```python
from build123d import *

# Parameters (mm, degrees)
F0_W     = 16
F0_H     = 10
F1_DEPTH = 30
F2_W     = 16
F2_H     = 7
F3_DEPTH = 8
F4_W     = 3.9
F4_H     = 5.5
F5_DEPTH = 8.4
F6_R     = 1.75
F7_DEPTH = 5
F8_F1_R  = 1
F8_F2_R  = 1
F8_F3_R  = 0.9999


# Not quite as in the source:
# - a fillet or chamfer is up to 0.001 mm smaller than in the source, because OpenCascade refuses the exact size
# - a feature names something its author has since deleted; it is built from what else it names


with BuildPart() as f1:
    # F0 (on Top) → F1 (new body)
    with BuildSketch(Plane.XY):
        Rectangle(F0_W, F0_H)
    extrude(amount=F1_DEPTH)

    # F2 (on face) → F3 (cut)
    with BuildSketch(Plane.XY.offset(30)):
        with Locations((0, -1.5)):
            Rectangle(F2_W, F2_H)
    extrude(amount=-F3_DEPTH, mode=Mode.SUBTRACT)

    # F4 (on face) → F5 (cut)
    with BuildSketch(Plane.XY.offset(22)):
        with Locations((-6.05, -0.75)):
            Rectangle(F4_W, F4_H)
        with Locations((6.05, -0.75)):
            Rectangle(F4_W, F4_H)
    extrude(amount=-F5_DEPTH, mode=Mode.SUBTRACT)

    # F6 (on face) → F7 (cut)
    with BuildSketch(Plane.XY.offset(22)):
        with Locations((0, -0.75)):
            Circle(F6_R)
    extrude(amount=-F7_DEPTH, mode=Mode.SUBTRACT)

    # F8: fillet of radius 1 on 13 edges, made by hand

    # F8_f1
    f8_f1_edges = [f1.edges().sort_by_distance(p)[0] for p in [
        (-4.1, -3.5, 17.8),
    ]]
    fillet(f8_f1_edges, radius=F8_F1_R)

    # F8_f2
    f8_f2_edges = [f1.edges().sort_by_distance(p)[0] for p in [
        (4.1, -0.75, 22),
        (-4.1, -0.25, 22),
        (6.05, -3.5, 22),
        (8, 3.5, 30),
        (-8, 3.5, 30),
        (0, 2, 30),
        (0, 5, 30),
        (-8, 2, 21.8),
        (8, 2, 21.8),
        (-4.3928932188, -3.2071067812, 22),
    ]]
    fillet(f8_f2_edges, radius=F8_F2_R)

    # F8_f3 (radius 1 in the source; OpenCascade refuses exactly that, so slightly less here)
    f8_f3_edges = [f1.edges().sort_by_distance(p)[0] for p in [
        (4.1, 2, 17.3),
        (-4.1, 2, 17.3),
        (0, 2, 22),
        (3.8071067812, 2, 21.7071067812),
        (-3.8071067812, 2, 21.7071067812),
    ]]
    fillet(f8_f3_edges, radius=F8_F3_R)


solid = f1.part
```
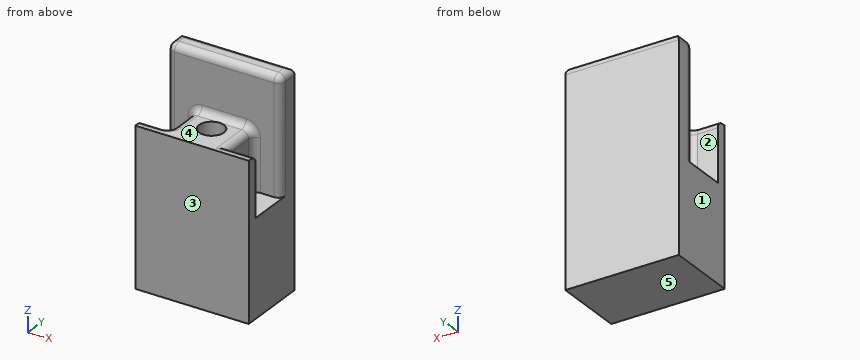
Source: CAD feature listing. Evaluate the final solid. Frame: model axes, mm. Face numbers are marked on the shaded views. A direction names the side the tool comes from. Round coordinates to 2 decimals unless told otherwise and drop trailing zeros. Loops run counter-clockwise (first coordinate to the right, second up) from the corner with the lowest first, then second, coordinate; pieces in that order, holes last. Notation, with made-up numbers: M -38.5,-24 L -0.5,-24 A12 ccw -0.5,-9 Z; hole C -12.75,-6 d9. An arc over 180 degrees is marked long. Use a Markdown table: item, result. Add a question column.
1. Section query A-A on y = -0.75. Return the cut outline in (x, z).
2. Reachability of the marked faces 4 and 5 from +Z, -Z, +X, -X, +Y, -Y: full face, straight path, thin tool, end or side. Return the list, or none.
3. Mould query, pull axis Y, two halves, no side actions, for the marked faces 1, 2 and 3. Classes: pulls with the +Y half, pulls with the -Y half, needs draft (parallel to the pull), parting line crosses it, or undercut.
4. Section query C-C on z = 24.25. Return the cut outline in (x, y), then the cut area to 3 significant figures.
5. Section query D-D on y = 1.5. Return the cut outline in (x, z), then the cut area to 3 significant figures.
6. Contact query for flat-ended pins moving along their axis: P1, Ø5, axis at x = 1, y = -2, coming from the +Z side; P2, Ø3, axis at x = 5, y = -1, coming from the +Z side; P3, Ø1.1, axis at y = 0, z = 16.5, coming from the -X side. Output: stop coordinate, or through.
7. Line query: line 1 (Y direction, x = -7, z = 20.75); line 2 (Y direction, x = 0, z = 18.95); line 3 (Z direction, x = 3, y = -0.25). Output: solid intervals per line, ascending.
Reported:
| question | item | result |
|---|---|---|
| 1 | outline | M -8,0 L 8,0 L 8,13.6 L 4.1,13.6 L 4.1,21 A1 ccw 3.1,22 L 1.75,22 L 1.75,17 L -1.75,17 L -1.75,22 L -3.1,22 A1 ccw -4.1,21 L -4.1,13.6 L -8,13.6 Z |
| 2 | face 4 | +Z, +X, -X, -Y |
| 2 | face 5 | -Z, +X, -X, +Y, -Y |
| 3 | face 1 | needs draft |
| 3 | face 2 | undercut |
| 3 | face 3 | pulls with the -Y half |
| 4 | outline | M -8,3 A1 ccw -7,2 L 7,2 A1 ccw 8,3 L 8,5 L -8,5 Z |
| 4 | area | 47.6 mm² |
| 5 | outline | M -8,0 L 8,0 L 8,13.6 L 4.23,13.6 L 4.23,21 A1.13 ccw 3.1,22.13 L -3.1,22.13 A1.13 ccw -4.23,21 L -4.23,13.6 L -8,13.6 Z |
| 5 | area | 289 mm² |
| 6 | P1 | stops at z = 22 |
| 6 | P2 | stops at z = 21.92 |
| 6 | P3 | stops at x = -4.1 |
| 7 | line 1 | y = -5 to -3.5, 2 to 5 |
| 7 | line 2 | y = -5 to -2.5, 1 to 5 |
| 7 | line 3 | z = 0 to 22 |
